The listing builds one solid part. Answer for the finished solid, in the listing's coordinates (mm). A direction names the side the tool comes from. Round coordinates to 2 decimals unless told otherwise and drop trailing zeros. Order: outer loops, then holes, each group sorted by start corner. A loop starts at its lowest first (then second) coordinate and runs counter-clockwise, first axis right, second up. Notation, with made-up numbers: M 36.25,28 L 57.25,28 A27 ccw 57.25,60 Z; hole C 61,52 d6. An arc over 180 degrees is marked long. Put each result on its own line as item: value. Start each with the question number.
1. The mould has two halves that part along Z. Classify faces 1 (the face through (0, 3, -17.462)), 2 (the face through (-12.7, 3, 5)), 3 (the face through (0.708, 3.131, 3.186)): +Z half, -Z half, draft (parallel to the pull), parting line (faces both ways), or undercut.
2. The part is cut by section C-C (x = -2.75). Give the vertices of the cut face in (y, z).
3. The part is cut by section B-B (y = 3). Give the vertices of the cut face in (x, z) (1 decimal), then the cut area to 3 significant figures.
4. The part is cut by section A-A (z = 0). Give the vertices of the cut face in (x, y).
5. Which of the six approach directions +Z, -Z, +X, -X, +Y, -Y give full straight-line access (tool end or side, diameter ignored) to faces 4 (the face through (-9, 3, -3.175)), 5 (the face through (3, 0, -3))?
6. Consider line 1 (Z direction, x = -8.75, y = 6) (1 decimal); line 2 (Z direction, x = -4.5, y = 4.5); line 3 (X direction, y = 2.5, z = -4). Determine where each line is inside the solid, lowest interval first.
from build123d import *

# Parameters (mm, degrees)
BOSS_EXTRUDE1_DEPTH         = 6.35
F_1_4_CLEARANCE_HOLE1_D     = 6.5278
F_1_4_CLEARANCE_HOLE1_DEPTH = 6.35
F_1_4_CLEARANCE_HOLE1_TIP   = 1.961148974


with BuildPart() as part:
    # Sketch2 → Boss-Extrude1 (new body)
    with BuildSketch(Plane(origin=(0, 0, 0), x_dir=(1, 0, 0), z_dir=(0, 1, 0))):
        Polygon((-12.7, 15.875), (-12.7, 17.4625), (12.7, 17.4625), (12.7, -12.7), (-12.7, -12.7), (-12.7, 3.175), (-5.7912, 3.175), (-5.7912, 3.683), (0, 3.683), (0, 15.367), (-5.7912, 15.367), (-5.7912, 15.875), align=None)
    extrude(amount=BOSS_EXTRUDE1_DEPTH)

    # 1/4 Clearance Hole1
    with Locations(Plane(origin=(0, 6.35, 0), x_dir=(1, 0, 0), z_dir=(0, 1, 0))):
        with Locations((0, 0)):
            Hole(F_1_4_CLEARANCE_HOLE1_D / 2, depth=F_1_4_CLEARANCE_HOLE1_DEPTH)
            with Locations((0, 0, -(F_1_4_CLEARANCE_HOLE1_DEPTH + F_1_4_CLEARANCE_HOLE1_TIP / 2))):  # 118° drill point
                Cone(0, F_1_4_CLEARANCE_HOLE1_D / 2, F_1_4_CLEARANCE_HOLE1_TIP, mode=Mode.SUBTRACT)


solid = part.part
Resolved:
1. face 1: -Z half
1. face 2: draft
1. face 3: undercut
2. outline: M 0,-17.46 L 6.35,-17.46 L 6.35,-15.37 L 0,-15.37 Z; M 0,-3.68 L 6.35,-3.68 L 6.35,-1.76 L 0,-1.76 Z; M 0,1.76 L 6.35,1.76 L 6.35,12.7 L 0,12.7 Z
3. outline: M -12.7,-17.5 L 12.7,-17.5 L 12.7,12.7 L -12.7,12.7 L -12.7,-3.2 L -5.8,-3.2 L -5.8,-3.7 L 0,-3.7 L 0,-15.4 L -5.8,-15.4 L -5.8,-15.9 L -12.7,-15.9 Z; hole C 0,0 d6.5
3. area: 577 mm2
4. outline: M -12.7,0 L -3.26,0 L -3.26,6.35 L -12.7,6.35 Z; M 3.26,0 L 12.7,0 L 12.7,6.35 L 3.26,6.35 Z
5. face 4: -X, +Y, -Y
5. face 5: +Z, -Z, +X, -X, -Y
6. line 1: -17.5 to -15.9, -3.2 to 12.7
6. line 2: -17.46 to -15.37, -3.68 to 12.7
6. line 3: 0 to 12.7
